Here's the drawing with two shaded views (mm, measured from the low corner). I have some questions. Coordinates: 2 decimals unless noted, no trailing zeros. Write each loop counter-clockwise with the first axis right and the second up, starting at its lowest first coordinate (ties: lowest second). Pieces come first, ordered by that corner, then holes.
Item 1: I want a section at C-C on x = 4.5. Please give me the cut outline in (y, z).
Item 2: For P1, Ø1.5, axis at x = 9, z = 19, coming from the +Y side; P2, Ø6, axis at x = 9.5, z = 9.5, coming from the +Y side; P3, Ø8, axis at x = 26.5, z = 8.5, coming from the -Y side; P4, Ø3, axis at x = 5, y = 20, coming from the +Z side, each with a flat end and sliding along its axis, tell me the tip position at first contact or that it passes through.
Item 3: I want a section at D-D on x = 13.5. Please give me the cut outline in (y, z).
Item 4: I want a section at A-A on z = 12. Please give me the cut outline in (x, y).
Item 5: If I drill on probe 1 along Y at (x, z) = (22, 11.75); probe 2 along Y at (x, z) = (5, 11.75), over which ranges is the centre line in solid material (lowest first)?
Item 6: Thinking about a two-plate mould opening in Y: for the marked faces 1, 2 and 3, which applies, +Y half, -Y half, draft (parallel to the pull), parting line (faces both ways), or undercut?
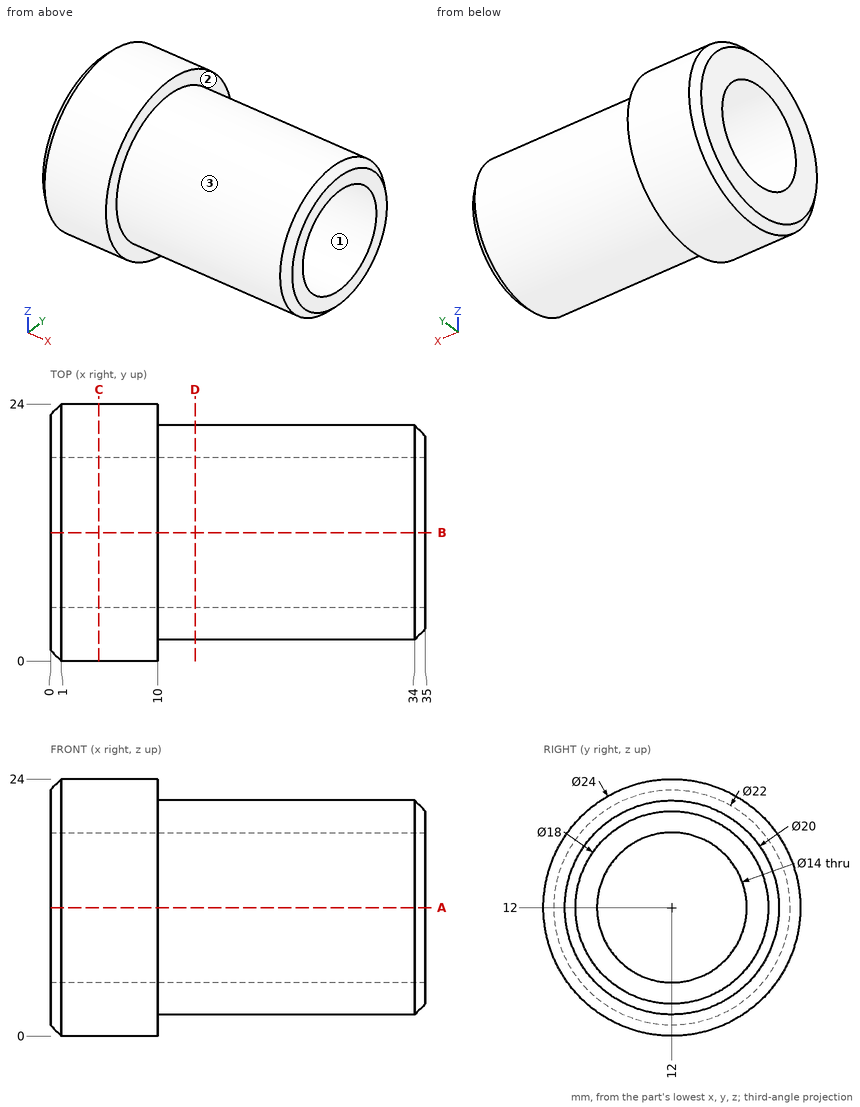
Response values:
1. outline: circle Ø24 at (12, 12); hole circle Ø14 at (12, 12)
2. P1: stops at y = 22.24
2. P2: stops at y = 24
2. P3: stops at y = 2
2. P4: stops at z = 22.09
3. outline: circle Ø20 at (12, 12); hole circle Ø14 at (12, 12)
4. outline: (0, 1) - (1, 0) - (10, 0) - (10, 2) - (34, 2) - (35, 3) - (35, 5) - (0, 5) - close; (0, 19) - (35, 19) - (35, 21) - (34, 22) - (10, 22) - (10, 24) - (1, 24) - (0, 23) - close
5. probe 1: y = 2 to 5, 19 to 22
5. probe 2: y = 0 to 5, 19 to 24
6. face 1: undercut
6. face 2: draft
6. face 3: parting line
